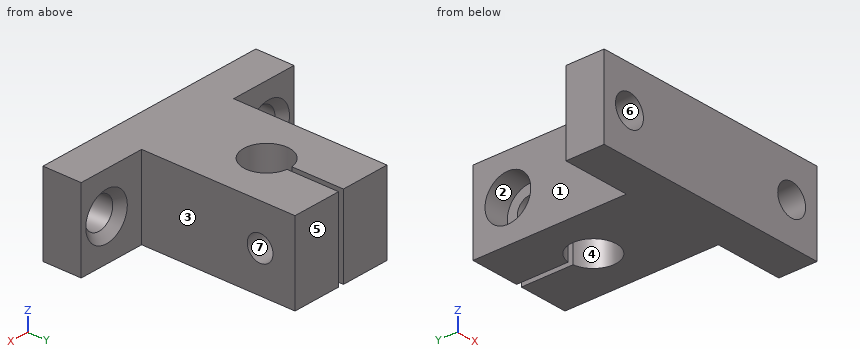
from build123d import *

# Parameters (mm, degrees)
BOSS_EXTRUDE1_DEPTH                                  = 7.15
CBORE_FOR_M4_HEX_SOCKET_HEAD_CAP_SCREW1_D            = 4.5
CBORE_FOR_M4_HEX_SOCKET_HEAD_CAP_SCREW1_CBORE_D      = 8
CBORE_FOR_M4_HEX_SOCKET_HEAD_CAP_SCREW1_CBORE_DEPTH  = 4.4
CSK_FOR_M5_HEX_SOCKET_COUNTERSUNK_CAP_SC_D           = 5.5
CSK_FOR_M5_HEX_SOCKET_COUNTERSUNK_CAP_SC_CSINK_D     = 8.2
CSK_FOR_M5_HEX_SOCKET_COUNTERSUNK_CAP_SC_CSINK_ANGLE = 90


with BuildPart() as part:
    # Sketch2 → Boss-Extrude1 (new, symmetric)
    with BuildSketch(Plane.XY):
        with BuildLine():
            Line((11.925, 6.68), (0, 6.68))
            Line((0, 6.68), (0, 0))
            Line((0, 0), (42, 0))
            Line((42, 0), (42, 6.68))
            Line((42, 6.68), (30.075, 6.68))
            Line((30.075, 6.68), (30.075, 33.5))
            Line((30.075, 33.5), (21.475, 33.5))
            Line((21.475, 33.5), (21.475, 24.471696741))
            ThreePointArc((21.475, 24.471696741), (21, 16.5), (20.525, 24.471696741))
            Line((20.525, 24.471696741), (20.525, 33.5))
            Line((20.525, 33.5), (11.925, 33.5))
            Line((11.925, 33.5), (11.925, 6.68))
        make_face()
    extrude(amount=BOSS_EXTRUDE1_DEPTH, both=True)

    # CBORE for M4 Hex Socket Head Cap Screw1 (through all)
    with Locations(Plane.ZY.offset(-11.925)):
        with Locations((0, 27.4)):
            CounterBoreHole(CBORE_FOR_M4_HEX_SOCKET_HEAD_CAP_SCREW1_D / 2, CBORE_FOR_M4_HEX_SOCKET_HEAD_CAP_SCREW1_CBORE_D / 2, CBORE_FOR_M4_HEX_SOCKET_HEAD_CAP_SCREW1_CBORE_DEPTH)

    # CSK for M5 Hex Socket Countersunk Cap Screw1 (through all)
    with Locations(Plane(origin=(0, 6.68, 0), x_dir=(1, 0, 0), z_dir=(0, 1, 0))):
        with Locations((5, 0), (37, 0)):
            CounterSinkHole(CSK_FOR_M5_HEX_SOCKET_COUNTERSUNK_CAP_SC_D / 2, CSK_FOR_M5_HEX_SOCKET_COUNTERSUNK_CAP_SC_CSINK_D / 2, counter_sink_angle=CSK_FOR_M5_HEX_SOCKET_COUNTERSUNK_CAP_SC_CSINK_ANGLE)


solid = part.part
Model file for the job. Use its own axes, mm. Face numbers are marked on the shaded views. A direction names the side the tool comes from. Round coordinates to 2 decimals unless told otherwise and drop trailing zeros. Loops run counter-clockwise (first coordinate to the right, second up) from the corner with the lowest first, then second, coordinate; pieces in that order, holes last. Notation, with made-up numbers: (52.25, 77) -> (90.25, 77) arc R6 cw to (90.25, 83) -> close; hole circle Ø10 at (-27.75, 84). An arc over 180 degrees is marked (long way). Answer as CSV lines item,"result". Start each with the question number.
1) Slice it at C-C (z = 0). State how many separate pieces and enclosed holes the cut face has, plus the area to 3 significant figures.
2) Pin check, flat tips, straight feed: P1, Ø7, axis at y = 28.5, z = 3.5, coming from the -X side (3 decimals); P2, Ø3, axis at y = 25.5, z = -4.5, coming from the +X side (3 decimals). Stop position of each tip, or through.
3) Mould opens along Y. For the marked faces 4, 5, 6 and 7 say: +Y half, -Y half, draft (parallel to the pull), parting line (faces both ways), or undercut.
4) Tool access for the marked faces 1, 2 and 3: list every direction of +Z, -Z, +X, -X, +Y, -Y with a clear straight run to the whole face (end or side of a thin tool).
5) Slice it at A-A (x = 37). List the corners of the cut face in (y, z).
6) Probe line 1 along Y through (x, z) = (13, 0); line 2 along Y through (x, z) = (24, -1); line 3 along Y through (x, z) = (18.5, 0). List the from-to ranges inside material, lowest first.
7) Slice it at D-D (x = 18). List the corners of the cut face in (y, z), plus the area to 3 significant figures.
8) Slice it at B-B (y = 20.5). List the corners of the cut face in (x, z) (3 decimals), plus the area to 3 significant figures.
Filled in:
1,separate pieces,"5"
1,enclosed holes,"0"
1,area,"539 mm2"
2,P1,"stops at x = 11.925"
2,P2,"stops at x = 30.075"
3,face 4,"undercut"
3,face 5,"+Y half"
3,face 6,"draft"
3,face 7,"undercut"
4,face 1,"+Z, -Z, -X, +Y"
4,face 2,"-X"
4,face 3,"+Z, -Z, +X, +Y"
5,outline,"(0, -7.15) -> (6.68, -7.15) -> (6.68, -4.1) -> (5.33, -2.75) -> (0, -2.75) -> close; (0, 2.75) -> (5.33, 2.75) -> (6.68, 4.1) -> (6.68, 7.15) -> (0, 7.15) -> close"
6,line 1,"y = 0 to 23.4, 31.4 to 33.5"
6,line 2,"y = 0 to 17.85, 23.15 to 25.38, 29.42 to 33.5"
6,line 3,"y = 0 to 17.38, 23.62 to 25.15, 29.65 to 33.5"
7,outline,"(0, -7.15) -> (17.85, -7.15) -> (17.85, 7.15) -> (0, 7.15) -> close; (23.15, -7.15) -> (33.5, -7.15) -> (33.5, 7.15) -> (23.15, 7.15) -> close; hole circle Ø4.5 at (27.4, 0)"
7,area,"387 mm2"
8,outline,"(11.925, -7.15) -> (17, -7.15) -> (17, 7.15) -> (11.925, 7.15) -> close; (25, -7.15) -> (30.075, -7.15) -> (30.075, 7.15) -> (25, 7.15) -> close"
8,area,"145 mm2"
